Check sheet for the drawn part. Datum: minimum x, y, z corner. Units: mm. A direction names the side the tool comes from. Round coordinates to 2 decimals unless told otherwise and drop trailing zeros. Loops run counter-clockwise (first coordinate to the right, second up) from the corner with the lowest first, then second, coordinate; pieces in that order, holes last. Notation, with made-up numbers: (89.25, 21.25) -> (141.25, 21.25) arc R16 ccw to (141.25, 33.25) -> close; hole circle Ø2 at (35, -16.75). An arc over 180 degrees is marked (long way). Return JSON: item names as keys, results as strings.
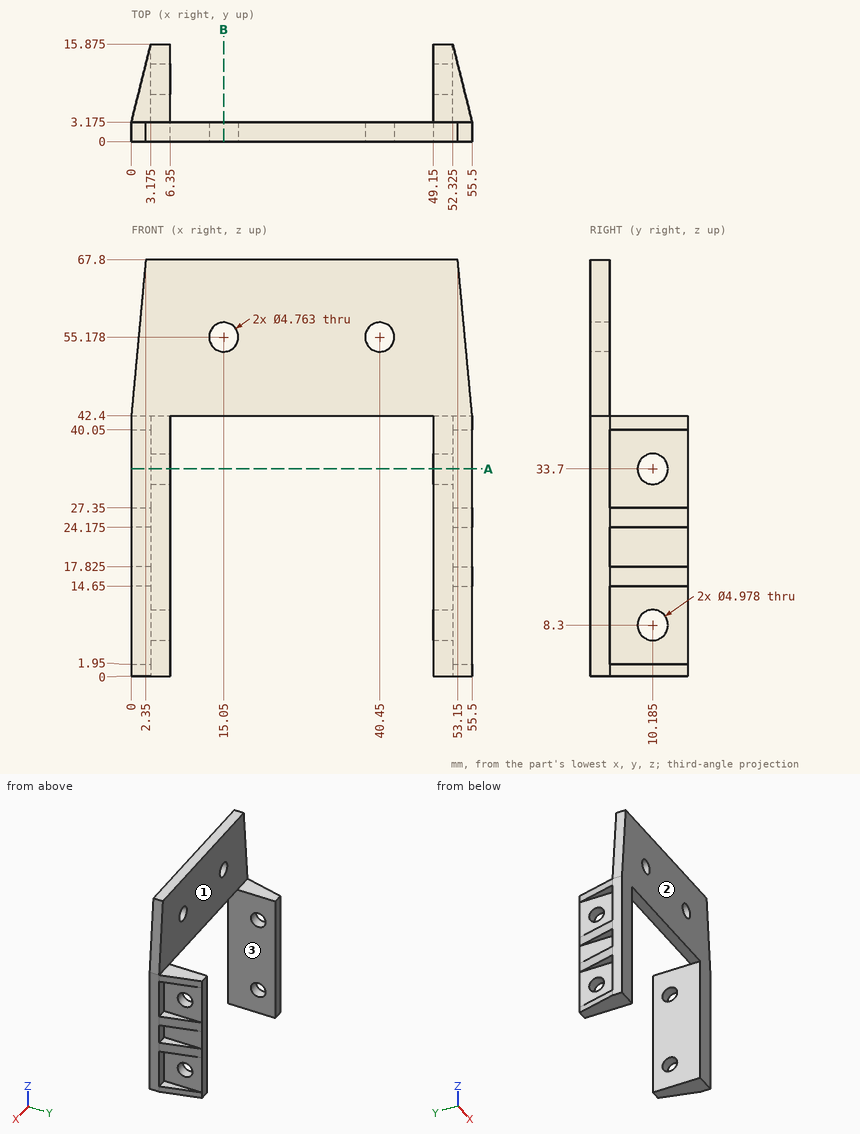
Q1. Section check B-B (x = 15.05). Record the boundary of the cut face in (y, z) (1 decimal).
Results list:
{"outline": "(0, 42.4) -> (3.2, 42.4) -> (3.2, 52.8) -> (0, 52.8) -> close; (0, 57.6) -> (3.2, 57.6) -> (3.2, 67.8) -> (0, 67.8) -> close"}
Q2. Material ranges on line 1 (Y direction, x = 4, z = 8) (1 decimal); line 2 (Z direction, x = 40.45, y = 0.75); line 3 (X direction, y = 2.5, z = 28), recorded low to high.
Results list:
{"line 1": "0 to 7.7, 12.7 to 15.9", "line 2": "42.4 to 52.8, 57.56 to 67.8", "line 3": "0 to 6.35, 49.15 to 55.5"}
Q3. Tool access check on the marked faces 1, 2 and 3. Record the directions out of +Z, -Z, +X, -X, +Y, -Y that give a thin tool (end or side, any length) a straight path to the whole face; none if there is none.
Results list:
{"face 1": "+Z, +X, -X, +Y", "face 2": "+Z, -Z, +X, -X, -Y", "face 3": "-Z, +Y, -Y"}
Q4. Section check A-A (z = 33.7). Count the separate pieces of the cut face and the enclosed holes in it.
Results list:
{"separate pieces": "4", "enclosed holes": "0"}
Q5. Go/stop test with flat-tipped pins: pin 1 (1 mm diameter, centred on x = 54.5, z = 21.5, fed in from +Y) (1 decimal); pin 2 (3.5 mm diameter, centred on x = 23, y = 2, fed in from -Z); pin 3 (6.5 mm diameter, centred on y = 10.19, z = 8.3, fed in from -X) (1 decimal). Record where each tip stops, or that it passes through.
Results list:
{"pin 1": "y = 3.2", "pin 2": "z = 42.4", "pin 3": "x = 3.2"}
